Autodesk Inventor part; units mm, degrees
ref_plane "YZ Plane" through (0, 0, 0) normal (1, 0, 0) x (0, 1, 0)
ref_plane "XZ Plane" through (0, 0, 0) normal (0, 1, 0) x (-1, 0, 0)
ref_plane "XY Plane" through (0, 0, 0) normal (0, 0, 1) x (1, 0, 0)
sketch "Skizze1" plane through (0, 0, 0) normal (0, 0, 1) x (1, 0, 0)
  line L0 (0, 0) -> (-22.3, 0)
  line L1 (-22.3, 0) -> (-22.3, 42)
  line L2 (-22.3, 42) -> (0, 42)
  line L3 (0, 42) -> (0, 0)
  line L4 (-19.3, 35) -> (-3, 35)
  line L5 (-3, 35) -> (-3, 33.4)
  line L6 (-3, 33.4) -> (-4.7, 33.4)
  line L7 (-4.7, 8.6) -> (-3, 8.6)
  line L8 (-3, 8.6) -> (-3, 7)
  line L9 (-3, 7) -> (-19.3, 7)
  line L10 (-19.3, 7) -> (-19.3, 35)
  line L11 (-4.7, 33.4) -> (-4.7, 8.6)
  line L12 (-11.15, 7) -> (-11.15, 0)
  line L13 (-11.15, 35) -> (-11.15, 42)
  dimension "d1" = 42
  dimension "d2" = 16.3
  dimension "d3" = 1.6
  dimension "d6" = 1.6
  dimension "d7" = 28
  dimension "d8" = 1.7
  dimension "d10" = 3
  dimension "d17" = 16.3
  dimension "d19" = 3
extrude "Extrusion1" add sketch "Skizze1" along normal blind 20 contours L0 L12 L9 L8 L7 L11 L6 L5 L4 L13 L2 L3 | L0 L1 L2 L13 L4 L10 L9 L12
sketch "Skizze2" plane through (0, 0, 20) normal (0, 0, 1) x (1, 0, 0)
  line L0 (0, 42) -> (-22.3, 42)
  line L1 (-22.3, 42) -> (0, 42)
  line L2 (0, 42) -> (0, 0)
  line L3 (0, 0) -> (-22.3, 0)
  line L4 (-22.3, 0) -> (-22.3, 42)
extrude "Extrusion2" add sketch "Skizze2" along normal blind 5
fillet "Rundung1" radius 3 12 edges at (-11.15, 0, 0) (-22.3, 21, 0) (0, 21, 0) (-11.15, 42, 0) (0, 21, 25) (0, 0, 12.5) (-11.15, 0, 25) (-22.3, 0, 12.5) (-22.3, 21, 25) (-11.15, 42, 25) (0, 42, 12.5) (-22.3, 42, 12.5)
properties part number "7.3 Endhalterung Schiene"
Here's how the part is built. I have some questions about the finished solid (model axes, mm). A direction names the side the tool comes from. Round coordinates to 2 decimals unless told otherwise and drop trailing zeros. Write each loop counter-clockwise with the first axis right and the second up, starting at its lowest first coordinate (ties: lowest second). Pieces come first, ordered by that corner, then holes.
1. For faces 5 (the flat face through (-4, 33.4, 10)), 6 (the flat face through (-11, 42, 12)), which set-ups out of +Z, -Z, +X, -X, +Y, -Y let a thin tool reach every point of the face, with its end or its side?
2. I need wall thicknesses on L1, parallel to Y at x = -12.5, z = 15.25; L2, parallel to X at y = 10, z = 4.75; L3, parallel to Y at x = -3.75, z = 2.5. Which ranges of each line are inside material? Lowest first, please.
3. If we mould it in two halves opening along X, with no side actions, what happens to faces 1 (the cylindrical face through (-11.04, 41.1, 0.86)), 2 (the flat face through (-19.3, 21, 10)), 3 (the flat face through (-22.3, 21, 12)), 4 (the cylindrical face through (-0.86, 41.1, 12.63))? For each: released by +X, released by -X, zero draft, split by the parting line, or undercut.
4. Suppose I cut it at C-C (x = -5.75). List the corners of the cut face in (y, z) for me, and give its area (3 significant figures).
5. Suppose I cut it at D-D (z = 23). List the corners of the cut face in (x, y) for me.
6. Suppose I cut it at A-A (z = 19). List the corners of the cut face in (x, y) for me, and give its area (3 significant figures).
Answer sheet:
1. face 5: -Z
1. face 6: +Z, -Z, +X, -X, +Y
2. L1: y = 0 to 7, 35 to 42
2. L2: x = -22.3 to -19.3, -4.7 to 0
2. L3: y = 0.04 to 7, 8.6 to 33.4, 35 to 41.96
3. face 1: zero draft
3. face 2: undercut
3. face 3: released by -X
3. face 4: released by +X
4. outline: (0, 3) arc R3 ccw to (3, 0) - (7, 0) - (7, 20) - (35, 20) - (35, 0) - (39, 0) arc R3 ccw to (42, 3) - (42, 22) arc R3 ccw to (39, 25) - (3, 25) arc R3 ccw to (0, 22) - close
4. area: 482 mm2
5. outline: (-22.13, 3) arc R2.83 ccw to (-19.3, 0.17) - (-3, 0.17) arc R2.83 ccw to (-0.17, 3) - (-0.17, 39) arc R2.83 ccw to (-3, 41.83) - (-19.3, 41.83) arc R2.83 ccw to (-22.13, 39) - close
6. outline: (-22.3, 3) arc R3 ccw to (-19.3, 0) - (-3, 0) arc R3 ccw to (0, 3) - (0, 39) arc R3 ccw to (-3, 42) - (-19.3, 42) arc R3 ccw to (-22.3, 39) - close; hole (-19.3, 7) - (-3, 7) - (-3, 8.6) - (-4.7, 8.6) - (-4.7, 33.4) - (-3, 33.4) - (-3, 35) - (-19.3, 35) - close
6. area: 515 mm2
